The listing builds one solid part. Answer for the finished solid, in the listing's coordinates (mm). A direction names the side the tool comes from. Coordinates: 2 decimals unless noted, no trailing zeros. Loops run counter-clockwise (first coordinate to the right, second up) from the corner with the lowest first, then second, coordinate; pieces in that order, holes last. Notation, with made-up numbers: M 8,33.25 L 64,33.25 A31 cw 64,61.25 Z; hole C 84,-15.75 d9. An arc over 180 degrees is marked long. Answer in a Markdown table with one row per item. Add a question column.
from build123d import *

# Parameters (mm, degrees)
F0_R            = 38.1
F1_DEPTH        = 76.2
F3_R            = 28.575
F4_DEPTH        = 6.35
F5_R            = 1.5
F6_DEPTH        = 50.8
F6_COPIES_COUNT = 2
F6_COPIES_ANGLE = 90
F2_R            = 15.875
F7_DEPTH        = 4.318
F7_FACE_R       = 15.875
F4_FACE_R       = 28.575
F9_R            = 38.1
F9_R_2          = 31.496
F10_DEPTH       = 6.35


# Not quite as in the source:
# - a pattern or mirror of a feature is missing from the dataset's text; its kind, count and spacing are read off the source's solid


with BuildPart() as f1:
    # F0 (on Top) → F1 (new body)
    with BuildSketch(Plane.XY):
        Circle(F0_R)
    extrude(amount=F1_DEPTH)

    # F3 (on face) → F4 (cut)
    with BuildSketch(Plane(origin=(0, 0, 0), x_dir=(1, 0, 0), z_dir=(0, 0, -1))):
        Circle(F3_R)
    extrude(amount=-F4_DEPTH, mode=Mode.SUBTRACT)

    # F5 (on Right) → F6 (cut)
    with BuildSketch(Plane.YZ):
        with Locations((0, 74.041)):
            Circle(F5_R)
    f6 = extrude(amount=-F6_DEPTH, mode=Mode.SUBTRACT)

    # F6_copies: F6 ×2 about axis
    f6_copies_axis = Axis((0, 0, 0), (0, 0, 1))
    for i in range(1, F6_COPIES_COUNT):
        add(f6.rotate(f6_copies_axis, i * F6_COPIES_ANGLE / (F6_COPIES_COUNT - 1)), mode=Mode.SUBTRACT)

    # F2 (on face) → F7 (cut)
    with BuildSketch(Plane.XY.offset(76.2)):
        Circle(F2_R)
    extrude(amount=-F7_DEPTH, mode=Mode.SUBTRACT)

    # F7_face (on face) → F8 section 0
    with BuildSketch(Plane.XY.offset(71.882)):
        Circle(F7_FACE_R)
    # F4_face (on face) → F8 section 1
    with BuildSketch(Plane(origin=(0, 0, 6.35), x_dir=(1, 0, 0), z_dir=(0, 0, -1))):
        Circle(F4_FACE_R)
    loft(mode=Mode.SUBTRACT)

    # F9 (on face) → F10 (cut)
    with BuildSketch(Plane(origin=(0, 0, 0), x_dir=(1, 0, 0), z_dir=(0, 0, -1))):
        Circle(F9_R)
        Circle(F9_R_2, mode=Mode.SUBTRACT)
    extrude(amount=-F10_DEPTH, mode=Mode.SUBTRACT)


solid = f1.part
(1) A cutting plane is placed at C-C (x = 33). Give the vertices of the cut face in (y, z).
(2) Straight lines are drawn through the part: line 1 (X direction, y = 0, z = 73) (3 decimals); line 2 (Z direction, x = 33.5, y = -17.5); line 3 (Y direction, x = 15.5, z = 29). For each, find the intervals that lie inside material, in ascending order.
(3) A cutting plane is placed at A-A (x = 0). Give the vertices of the cut face in (y, z) (3 decimals).
(4) Each of these flat-tipped pins is pushed along its axis until it touches: pin 1 (6 mm diameter, centred on x = 10, z = 42, fed in from +Y); pin 2 (1 mm diameter, centred on x = 29.5, z = 48.5, fed in from +Y); pin 3 (2.5 mm diameter, centred on x = 0, z = 74.041, fed in from -Y). Where does it stop, or does it pass through?
(5) For faces 4 (the face through (-6.828, 30.747, 3.131)), 5 (the face through (-26.8, 0.69, 72.71)), 6 (the face through (-0.69, -26.8, 72.71)), determine the directions among +Z, -Z, +X, -X, +Y, -Y from which every point of the face is accessible in a straight line to the end or side of a thin tool.
(6) The mould has two halves that part along Y. Classify faces 1 (the face through (-30.235, -23.183, 40.786)), 2 (the face through (-28.547, -1.256, 3.131)), 3 (the face through (-14.3, -28.4, 6.35)): released by +Y, released by -Y, zero draft, split by the parting line, or undercut.
(7) A cutting plane is placed at B-B (y = 0). State how many separate pieces and enclosed holes the cut face has, plus the area to 3 significant figures.
Solved:
| question | item | result |
|---|---|---|
| 1 | outline | M -19.04,6.35 L 19.04,6.35 L 19.04,76.2 L -19.04,76.2 Z |
| 2 | line 1 | x = 15.875 to 38.1 |
| 2 | line 2 | z = 6.35 to 76.2 |
| 2 | line 3 | y = -34.8 to -18.57, 18.57 to 34.8 |
| 3 | outline | M -38.1,6.35 L -31.496,6.35 L -31.496,0 L -28.575,0 L -28.575,6.35 L -15.875,71.882 L -15.875,72.541 L -38.1,72.541 Z; M -38.1,75.541 L -15.875,75.541 L -15.875,76.2 L -38.1,76.2 Z; M 15.875,71.882 L 28.575,6.35 L 28.575,0 L 31.496,0 L 31.496,6.35 L 38.1,6.35 L 38.1,76.2 L 15.875,76.2 Z |
| 4 | pin 1 | stops at y = 37.45 |
| 4 | pin 2 | stops at y = 24.71 |
| 4 | pin 3 | stops at y = 15.83 |
| 5 | face 4 | -Z |
| 5 | face 5 | -X |
| 5 | face 6 | -Y |
| 6 | face 1 | split by the parting line |
| 6 | face 2 | undercut |
| 6 | face 3 | zero draft |
| 7 | separate pieces | 3 |
| 7 | enclosed holes | 0 |
| 7 | area | 2,240 mm² |
